```python
from build123d import *

# Parameters (mm, degrees)
F1_DEPTH = 6


with BuildPart() as f1:
    # F0 (on Front) → F1 (new body)
    with BuildSketch(Plane.XZ):
        Polygon((0, 22.677863), (0, 58.5), (-21, 58.5), (-21, 63.5), (0, 63.5), (0, 63.75), (0, 122.5), (-21, 122.5), (-21, 127.5), (-0.465679, 127.5), (-0.465679, 173.380539), (-128.12072, 173.380539), (-26.326123, 6.608847), align=None)
        Polygon((0, 250), (-128.12072, 173.380539), (-0.465679, 173.380539), (-0.465679, 186.25), (-21, 186.25), (-21, 191.25), (0, 191.25), align=None)
    extrude(amount=F1_DEPTH)


solid = f1.part
```
Model file for the job. Use its own axes, mm. A direction names the side the tool comes from. Coordinates: 2 decimals unless noted, no trailing zeros. Loops run counter-clockwise (first coordinate to the right, second up) from the corner with the lowest first, then second, coordinate; pieces in that order, holes last. Notation, with made-up numbers: (75, 13.25) - (102, 13.25) arc R14 cw to (102, 17.25) - close; hole circle Ø11 at (-21.75, 67.25). An arc over 180 degrees is marked (long way). Write item = value, one per line. Start each with the question number.
Item 1: Saw through at C-C, the plane z = 101. List the corners of the cut face in (x, y).
Item 2: Saw through at B-B, the plane x = -117. List the corners of the cut face in (y, z), then the cut area to 3 significant figures.
Item 3: Drop flat-ended pins along their axis: pin 1 Ø1 at (x, y) = (-34.5, -1) entering from -Z; pin 2 Ø1.8 at (x, y) = (-5.5, -4) entering from -Z; pin 3 Ø1 at (x, y) = (-24, -4.5) entering from +Z. Give the stop position or say it passes through.
Item 4: Wall check: probe 1 along Z at (x, y) = (-20, -0.65); probe 2 along X at (y, z) = (-3.5, 239.5); probe 3 along Z at (x, y) = (-67, -5.2). Give the ranges that are in metal, low to high. Write a range as [from, to].
Item 5: Pull direction Z, two halves, no side cores. Call faces 3 (the face through (0, -3, 220)), 4 (the face through (-63.16, -2.96, 212.23)), 5 (the face through (-11, -3, 63.5)), 6 (the face through (-21, -3, 189)): +Z half, -Z half, draft (parallel to the pull), parting line (faces both ways), or undercut.
Item 6: Saw through at A-A, the plane y = -4.45. List the corners of the cut face in (x, z), then the cut area to 3 significant figures.
Item 7: 3-axis set-ups, long thin cutter, end or side, ignore diameter. For faces 1 (the face through (-0.466, -3, 156)), 2 (the face through (-77.936, -2.958, 91.162)): which of +Z, -Z, +X, -X, +Y, -Y reach the whole face in a straight line?
Answers:
q1.outline = (-83.94, -6) - (0, -6) - (0, 0) - (-83.94, 0) - close
q2.outline = (-6, 155.16) - (0, 155.16) - (0, 180.03) - (-6, 180.03) - close
q2.area = 149 mm2
q3.pin_1 = 19.18
q3.pin_2 = 18.77
q3.pin_3 = 235.95
q4.probe_1 = [10.47, 58.5], [63.5, 122.5], [127.5, 186.25], [191.25, 238.04]
q4.probe_2 = [-17.56, 0]
q4.probe_3 = [73.25, 209.93]
q5.face_3 = draft
q5.face_4 = +Z half
q5.face_5 = undercut
q5.face_6 = undercut
q6.outline = (-128.12, 173.38) - (-26.33, 6.61) - (0, 22.68) - (0, 58.5) - (-21, 58.5) - (-21, 63.5) - (0, 63.5) - (0, 122.5) - (-21, 122.5) - (-21, 127.5) - (-0.47, 127.5) - (-0.47, 186.25) - (-21, 186.25) - (-21, 191.25) - (0, 191.25) - (0, 250) - close
q6.area = 17,200 mm2
q7.face_1 = +X, +Y, -Y
q7.face_2 = -Z, -X, +Y, -Y
